Read the model definition and answer for the solid it produces. Units are mm, in the model's axes. A direction names the side the tool comes from. Give positions to 0.01 mm unless a question says otherwise; leave off trailing zeros. Write each loop counter-clockwise with the first axis right and the second up, starting at its lowest first coordinate (ties: lowest second). Pieces come first, ordered by that corner, then holes. Notation, with made-up numbers: (72.5, 83) -> (80.5, 83) arc R29 cw to (80.5, 119) -> close; hole circle Ø9 at (-3, 35). An arc over 180 degrees is marked (long way). Write item = value, one per line.
from build123d import *

# Parameters (mm, degrees)
EXTRUDE_2_DEPTH     = 40
SKETCH_3_R          = 1.75
CUT_EXTRUDE_1_DEPTH = 5
FILLET_1_R          = 0.5
SKETCH_2_R          = 1.5
CUT_EXTRUDE_2_DEPTH = 5


with BuildPart() as part:
    # ｽｹｯﾁ1 → ﾎﾞｽ - 押し出し2 (new body)
    with BuildSketch(Plane.XY):
        Polygon((3, 0), (1.5, 2.598076211), (-1.5, 2.598076211), (-3, 0), (-1.5, -2.598076211), (1.5, -2.598076211), align=None)
    extrude(amount=EXTRUDE_2_DEPTH)

    # ｽｹｯﾁ3 → ｶｯﾄ - 押し出し1 (cut)
    with BuildSketch(Plane(origin=(0, 0, 0), x_dir=(-1, 0, 0), z_dir=(0, 0, -1))):
        Circle(SKETCH_3_R)
    extrude(amount=-CUT_EXTRUDE_1_DEPTH, mode=Mode.SUBTRACT)

    # ﾌｨﾚｯﾄ1
    fillet_1_edges = [part.edges().sort_by_distance(p)[0] for p in [
        (0, 2.598076211, 40),
        (-2.25, 1.299038106, 40),
        (-2.25, -1.299038106, 40),
        (0, -2.598076211, 40),
        (2.25, -1.299038106, 40),
        (0, -2.598076211, 0),
        (-2.25, -1.299038106, 0),
        (-2.25, 1.299038106, 0),
        (2.25, 1.299038106, 40),
        (0, 2.598076211, 0),
        (2.25, 1.299038106, 0),
        (2.25, -1.299038106, 0),
    ]]
    fillet(fillet_1_edges, radius=FILLET_1_R)

    # ｽｹｯﾁ2 → ｶｯﾄ - 押し出し2 (cut)
    with BuildSketch(Plane.XY.offset(40)):
        Circle(SKETCH_2_R)
    extrude(amount=-CUT_EXTRUDE_2_DEPTH, mode=Mode.SUBTRACT)


solid = part.part
(1) The part is cut by section A-A on z = 21.5. Determine the outline of the cut face in (x, y).
Checks:
outline = (-3, 0) -> (-1.5, -2.6) -> (1.5, -2.6) -> (3, 0) -> (1.5, 2.6) -> (-1.5, 2.6) -> close
(2) Consider L1, parallel to Y at x = 0, z = 1.9; L2, parallel to Y at x = 0, z = 37.45; L3, parallel to X at y = -1.55, z = 26. Determine where each line is inside the solid, lowest interval first.
Checks:
L1 = -2.6 to -1.75, 1.75 to 2.6
L2 = -2.6 to -1.5, 1.5 to 2.6
L3 = -2.11 to 2.11
(3) Given P1, Ø1.5, axis at x = 0.5, y = 0.5, coming from the -Z side; P2, Ø2, axis at y = 1.5, z = 5.5, coming from the +X side; P3, Ø1.5, axis at y = 1, z = 33, coming from the -X side, each flat-ended and moving along its own axis, determine where each tip first touches the part or whether it passes through.
Checks:
P1 = 5
P2 = 2.71
P3 = -2.86
(4) A tool of negligible diameter and unlimited length cuts with its end or side. For faces 1 (the flat face through (0, 0, 35)), 2 (the flat face through (0, 0, 5)), 3 (the flat face through (-2.24, 1.32, 19.73)), from which of +Z, -Z, +X, -X, +Y, -Y can it reach the whole face along a straight path? Write none if from no direction.
Checks:
face_1 = +Z
face_2 = -Z
face_3 = +Z, -Z, -X, +Y
(5) For a pull along X with two mould halves and no side action, classify faces 4 (the cylindrical face through (-1.5, 0.07, 37.53)), 5 (the cylindrical face through (-2.13, 1.206, 39.857)), 6 (the cylindrical face through (2.116, 1.246, 0.15)) as released by +X, released by -X, zero draft, split by the parting line, or undercut.
Checks:
face_4 = undercut
face_5 = released by -X
face_6 = released by +X
(6) The part is cut by section B-B on x = -0.75. Determine the outline of the cut face in (y, z), plus the area to 3 significant figures.
Checks:
outline = (-2.6, 0.5) arc R0.5 ccw to (-2.1, 0) -> (-1.58, 0) -> (-1.58, 5) -> (1.58, 5) -> (1.58, 0) -> (2.1, 0) arc R0.5 ccw to (2.6, 0.5) -> (2.6, 39.5) arc R0.5 ccw to (2.1, 40) -> (1.3, 40) -> (1.3, 35) -> (-1.3, 35) -> (-1.3, 40) -> (-2.1, 40) arc R0.5 ccw to (-2.6, 39.5) -> close
area = 179 mm²
